Geometry: see drawing. Coordinates: mm, zero at the bounding-box minimum. A direction names the side the tool comes from. Give positions to 0.01 mm unless a question says otherwise; leave off trailing zeros. Order: outer loops, then holes, each group sorted by start corner. A loop starts at its lowest first (then second) coordinate and runs counter-clockwise, first axis right, second up. Notation, with made-up numbers: M 70.25,31.5 L 118.25,31.5 A29 cw 118.25,65.5 Z; hole C -20.75,87 d5. An arc over 180 degrees is marked long. Write item = value, one per line. Start each with the question number.
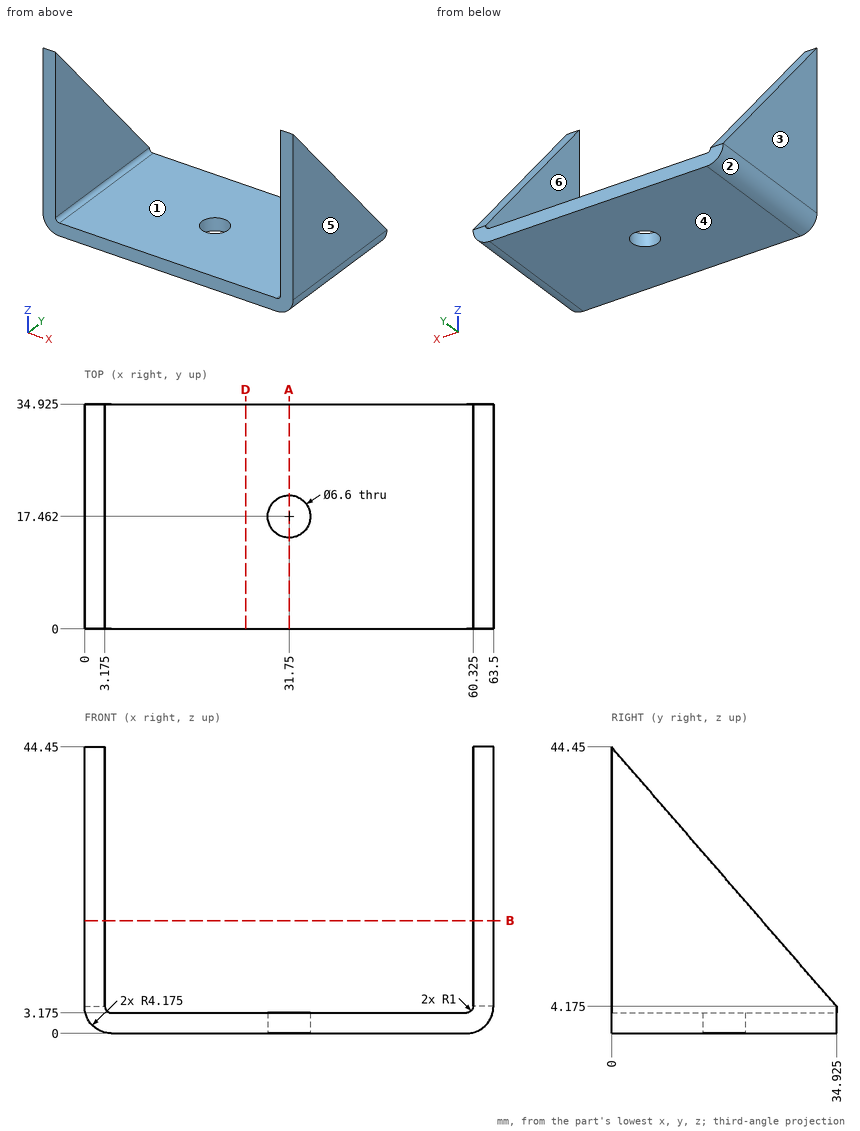
1) Draft query along X for the marked faces 3, 4, 5 and 6. Return one class per face: pulls with the +X half, pulls with the -X half, needs draft (parallel to the pull), parting line crosses it, or undercut.
2) Access query for the marked faces 1 and 2. Directions: +Z, -Z, +X, -X, +Y, -Y. A direction counts if a zero-diameter tool reaches every point of the face in a straight line with its end or side. Return the directions, or none.
3) Cut plane D-D (x = 25). Return loops of the section in (y, z) (1 decimal).
4) Cut plane B-B (z = 17.5). Return loops of the section in (x, y) (1 decimal).
5) Ray query, L1, parallel to Y at x = 31.75, z = 2.55 (1 decimal); L2, parallel to X at y = 10.5, z = 6 (1 decimal); L3, parallel to Z at x = 53, y = 23 (1 decimal). Return the intervals inside material, ascending.
6) Cut plane A-A (x = 31.75). Return loops of the section in (y, z) (1 decimal).
7) Pin query (flat end, axial travel): pin 1 Ø6 at (y, z) = (9.5, 39.5) entering from +X. Return the tip coordinate at first contact, or that it passes through.
Reply:
q1.face_3 = pulls with the -X half
q1.face_4 = needs draft
q1.face_5 = pulls with the +X half
q1.face_6 = undercut
q2.face_1 = +Z, +Y, -Y
q2.face_2 = -Z, -X, +Y, -Y
q3.outline = M 0,0 L 34.9,0 L 34.9,3.2 L 0,3.2 Z
q4.outline = M 0,0 L 3.2,0 L 3.2,23.4 L 0,23.4 Z; M 60.3,0 L 63.5,0 L 63.5,23.4 L 60.3,23.4 Z
q5.L1 = 0 to 14.2, 20.8 to 34.9
q5.L2 = 0 to 3.2, 60.3 to 63.5
q5.L3 = 0 to 3.2
q6.outline = M 0,0 L 14.2,0 L 14.2,3.2 L 0,3.2 Z; M 20.8,0 L 34.9,0 L 34.9,3.2 L 20.8,3.2 Z
q7.pin_1 = through
